```python
from build123d import *

# Parameters (mm, degrees)
SKETCH_1_R          = 50
EXTRUDE_1_DEPTH     = 6
SKETCH_2_R          = 1.75
CUT_EXTRUDE_1_DEPTH = 24
SKETCH_4_R          = 3
CUT_EXTRUDE_2_DEPTH = 24
SKETCH_5_R          = 11.5
CUT_EXTRUDE_3_DEPTH = 3
SKETCH_6_R          = 1.75
CUT_EXTRUDE_4_DEPTH = 37
SKETCH_7_R          = 3
CUT_EXTRUDE_5_DEPTH = 3
SKETCH_8_R          = 3.5
CUT_EXTRUDE_6_DEPTH = 3


with BuildPart() as part:
    # 草图1 → 凸台-拉伸1 (new body)
    with BuildSketch(Plane(origin=(0, 0, 0), x_dir=(1, 0, 0), z_dir=(0, 1, 0))):
        with Locations(Location((0, 0, 0), (0, 0, 270))):
            Circle(SKETCH_1_R)
    extrude(amount=EXTRUDE_1_DEPTH)

    # 草图2 → 切除-拉伸1 (cut)
    with BuildSketch(Plane(origin=(0, 6, 0), x_dir=(1, 0, 0), z_dir=(0, 1, 0))):
        with Locations(Location((0, 40, 0), (0, 0, 270))):
            Circle(SKETCH_2_R)
        with Locations(Location((40, 0, 0), (0, 0, 270))):
            Circle(SKETCH_2_R)
        with Locations(Location((-40, 0, 0), (0, 0, 270))):
            Circle(SKETCH_2_R)
    extrude(amount=-CUT_EXTRUDE_1_DEPTH, mode=Mode.SUBTRACT)

    # 草图4 → 切除-拉伸2 (cut)
    with BuildSketch(Plane.XZ):
        with Locations(Location((0, 28.284271247, 0), (0, 0, 270))):
            Circle(SKETCH_4_R)
    extrude(amount=-CUT_EXTRUDE_2_DEPTH, mode=Mode.SUBTRACT)

    # 草图5 → 切除-拉伸3 (cut)
    with BuildSketch(Plane(origin=(0, 6, 0), x_dir=(1, 0, 0), z_dir=(0, 1, 0))):
        with Locations(Location((0, -28.284271247, 0), (0, 0, 270))):
            Circle(SKETCH_5_R)
    extrude(amount=-CUT_EXTRUDE_3_DEPTH, mode=Mode.SUBTRACT)

    # 草图6 → 切除-拉伸4 (cut)
    with BuildSketch(Plane(origin=(0, 6, 0), x_dir=(1, 0, 0), z_dir=(0, 1, 0))):
        with Locations(Location((15.494, -12.790271247, 0), (0, 0, 270))):
            Circle(SKETCH_6_R)
        with Locations(Location((15.494, -43.778271247, 0), (0, 0, 270))):
            Circle(SKETCH_6_R)
        with Locations(Location((-15.494, -43.778271247, 0), (0, 0, 270))):
            Circle(SKETCH_6_R)
        with Locations(Location((-15.494, -12.790271247, 0), (0, 0, 270))):
            Circle(SKETCH_6_R)
    extrude(amount=-CUT_EXTRUDE_4_DEPTH, mode=Mode.SUBTRACT)

    # 草图7 → 切除-拉伸5 (cut)
    with BuildSketch(Plane.XZ):
        with Locations(Location((15.494, 43.778271247, 0), (0, 0, 270))):
            Circle(SKETCH_7_R)
        with Locations(Location((15.494, 12.790271247, 0), (0, 0, 270))):
            Circle(SKETCH_7_R)
        with Locations(Location((-15.494, 12.790271247, 0), (0, 0, 270))):
            Circle(SKETCH_7_R)
        with Locations(Location((-15.494, 43.778271247, 0), (0, 0, 270))):
            Circle(SKETCH_7_R)
    extrude(amount=-CUT_EXTRUDE_5_DEPTH, mode=Mode.SUBTRACT)

    # 草图8 → 切除-拉伸6 (cut)
    with BuildSketch(Plane(origin=(0, 6, 0), x_dir=(1, 0, 0), z_dir=(0, 1, 0))):
        with Locations(Location((0, 40, 0), (0, 0, 270))):
            Circle(SKETCH_8_R)
        with Locations(Location((-40, 0, 0), (0, 0, 270))):
            Circle(SKETCH_8_R)
        with Locations(Location((40, 0, 0), (0, 0, 270))):
            Circle(SKETCH_8_R)
    extrude(amount=-CUT_EXTRUDE_6_DEPTH, mode=Mode.SUBTRACT)


solid = part.part
```
Could you check a few things on this model? Use its own coordinates, in mm. A direction names the side the tool comes from. Coordinates: 2 decimals unless noted, no trailing zeros. Order: outer loops, then holes, each group sorted by start corner. A loop starts at its lowest first (then second) coordinate and runs counter-clockwise, first axis right, second up. Notation, with made-up numbers: M 9.5,-22.75 L 68.5,-22.75 A24 ccw 68.5,5.25 Z; hole C 35.25,-3 d10. An arc over 180 degrees is marked long. Use a Markdown table: item, result. Add a question column.
Q1. I want a section at C-C on z = -40. List the corners of the cut face in (x, y) for me, then the cut area to 4 significant figures.
Q2. We'd pull the mould along Z, two halves only. Please class faces 1 (the flat face through (1, 0, -1)), 2 (the cylindrical face through (0.901, 1.479, 25.423)): pulls with the +Z half, pulls with the -Z half, needs draft (parallel to the pull), parting line crosses it, or undercut.
Q3. I'm going to push flat-ended pins straight in: pin 1 (1.5 mm diameter, centred on y = 4, z = -33.5, fed in from -X); pin 2 (11 mm diameter, centred on x = 0, z = -40, fed in from -Y); pin 3 (1.5 mm diameter, centred on x = -24.5, y = 2.5, fed in from -Z); pin 4 (1 mm diameter, centred on y = 5, z = 0, fed in from -X). Where does each tip first touch, or does it pass through?
Q4. Which directions (+Z, -Z, +X, -X, +Y, -Y) give clear straight access to the entire face, cutting with the end or side of a thin tool? Please do faces 3 (the cylindrical face through (-41.71, 1.52, -0.38)), 4 (the cylindrical face through (17.522, 1.479, 15.001)), 5 (the flat face through (-38, 3, 1)).
Q5. I want a section at A-A on x = -40. List the corners of the cut face in (y, z) for me, then the cut area to 4 significant figures.
Q6. I want a section at B-B on z = 0. List the corners of the cut face in (x, y) for me, then the cut area to 3 significant figures.
Q7. If I drill on L1, parallel to X at y = 1.9, z = 0; L2, parallel to Z at x = 18, y = 2.65; L3, parallel to Z at x = 13, y = 1.15, over which ranges is the centre line in solid material (lowest first)?
Q8. I want a section at D-D on y = 4.4. Give the number of separate pieces and of enclosed holes in the cut face, then the cut area to 3 significant figures.
Checked values:
| question | item | result |
|---|---|---|
| 1 | outline | M -30,0 L -1.75,0 L -1.75,3 L -3.5,3 L -3.5,6 L -30,6 Z; M 1.75,0 L 30,0 L 30,6 L 3.5,6 L 3.5,3 L 1.75,3 Z |
| 1 | area | 328.5 mm² |
| 2 | face 1 | needs draft |
| 2 | face 2 | undercut |
| 3 | pin 1 | x = -37.78 |
| 3 | pin 2 | y = 0 |
| 3 | pin 3 | z = -44 |
| 3 | pin 4 | x = -50 |
| 4 | face 3 | +Y, -Y |
| 4 | face 4 | -Y |
| 4 | face 5 | +Y |
| 5 | outline | M 0,-30 L 6,-30 L 6,-3.5 L 3,-3.5 L 3,-1.75 L 0,-1.75 Z; M 0,1.75 L 3,1.75 L 3,3.5 L 6,3.5 L 6,30 L 0,30 Z |
| 5 | area | 328.5 mm² |
| 6 | outline | M -50,0 L -41.75,0 L -41.75,3 L -43.5,3 L -43.5,6 L -50,6 Z; M -38.25,0 L 38.25,0 L 38.25,3 L 36.5,3 L 36.5,6 L -36.5,6 L -36.5,3 L -38.25,3 Z; M 41.75,0 L 50,0 L 50,6 L 43.5,6 L 43.5,3 L 41.75,3 Z |
| 6 | area | 537 mm² |
| 7 | L1 | -50 to -41.75, -38.25 to 38.25, 41.75 to 50 |
| 7 | L2 | -46.65 to 11.14, 14.44 to 42.13, 45.43 to 46.65 |
| 7 | L3 | -48.28 to 11.12, 14.46 to 42.11, 45.45 to 48.28 |
| 8 | separate pieces | 1 |
| 8 | enclosed holes | 8 |
| 8 | area | 7,280 mm² |
